Check sheet for the modelled part. Datum: model origin and axes. Units: mm. A direction names the side the tool comes from. Round coordinates to 2 decimals unless told otherwise and drop trailing zeros. Loops run counter-clockwise (first coordinate to the right, second up) from the corner with the lowest first, then second, coordinate; pieces in that order, holes last. Notation, with made-up numbers: (80, 40) - (127, 40) arc R21 ccw to (127, 64) - close; hole circle Ø2 at (-0.75, -39.75). An arc over 180 degrees is marked (long way). Return JSON: item names as keys, results as strings.
from build123d import *

# Parameters (mm, degrees)
EXTRUSION1_DEPTH = 115
ESQUISSE6_R      = 1.5
ESQUISSE6_W      = 11.044450352
ESQUISSE6_H      = 20
EXTRUSION2_DEPTH = 120


with BuildPart() as part:
    # Esquisse5 → Extrusion1 (new body)
    with BuildSketch(Plane(origin=(0, 0, 0), x_dir=(1, 0, 0), z_dir=(0, 1, 0))):
        with BuildLine():
            Line((-11.982008115, -35.006163479), (-12.953522286, -37.844501059))
            ThreePointArc((-12.953522286, -37.844501059), (-37.203278989, -14.694081546), (-35.317903714, 18.778862511))
            Line((-35.317903714, 18.778862511), (-32.669060936, 17.370447823))
            ThreePointArc((-32.669060936, 17.370447823), (-34.413033065, -13.59202543), (-11.982008115, -35.006163479))
        make_face()
    extrude(amount=EXTRUSION1_DEPTH)

    # Esquisse6 → Extrusion2 (cut)
    with BuildSketch(Plane(origin=(0, 0, 0), x_dir=(0, 0, -1), z_dir=(1, 0, 0))):
        with Locations((0, 94)):
            Circle(ESQUISSE6_R)
        with Locations((0, 87)):
            Circle(ESQUISSE6_R)
        with Locations((0, 15)):
            Circle(ESQUISSE6_R)
        with Locations((0, 22)):
            Circle(ESQUISSE6_R)
        with Locations((23.022225176, 59)):
            Rectangle(ESQUISSE6_W, ESQUISSE6_H)
    extrude(amount=-EXTRUSION2_DEPTH, mode=Mode.SUBTRACT)


solid = part.part
Q1. Tool access check on faces 1 (the face through (-12.461, 56.695, 36.405)), 2 (the face through (-34, 59, -17.5)). Record the directions out of +Z, -Z, +X, -X, +Y, -Y that give a thin tool (end or side, any length) a straight path to the whole face; none if there is none.
Answer key:
{"face 1": "+Z, +X, +Y, -Y", "face 2": "-Z, +X, -X"}
Q2. Sectioned sample at A-A (z = 0). Enter the section's corners in (x, y).
Answer key:
{"outline": "(-40, 0) - (-37, 0) - (-37, 13.5) - (-40, 13.5) - close; (-40, 16.5) - (-37, 16.5) - (-37, 20.5) - (-40, 20.5) - close; (-40, 23.5) - (-37, 23.5) - (-37, 85.5) - (-40, 85.5) - close; (-40, 88.5) - (-37, 88.5) - (-37, 92.5) - (-40, 92.5) - close; (-40, 95.5) - (-37, 95.5) - (-37, 115) - (-40, 115) - close"}
Q3. Sectioned sample at D-D (x = -28). Enter the section's corners in (y, z), plus the area to 3 significant figures.
Answer key:
{"outline": "(0, 24.19) - (115, 24.19) - (115, 28.57) - (0, 28.57) - close", "area": "504 mm²"}
Q4. Draft check along Y on faces 3 (the face through (-35, 0, 14)), 4 (the face through (-38.463, 95.487, 0.195)), 5 (the face through (-34.012, 43.917, -18.085)). Enter one of: released by +Y, released by -Y, zero draft, split by the parting line, or undercut.
Answer key:
{"face 3": "released by -Y", "face 4": "undercut", "face 5": "zero draft"}
Q5. Sectioned sample at B-B (y = 87). Enter the section's corners in (x, z), plus the area to 3 significant figures.
Answer key:
{"outline": "(-39.97, -1.5) arc R40 ccw to (-35.32, -18.78) - (-32.67, -17.37) arc R37 cw to (-36.97, -1.5) - close; (-39.97, 1.5) - (-36.97, 1.5) arc R37 cw to (-11.98, 35.01) - (-12.95, 37.84) arc R40 ccw to start", "area": "191 mm²"}
Q6. Depth check by flat-ended pin: P1, Ø2.5, axis at y = 87, z = 0, coming from the +X side (3 decimals); P2, Ø3.5, axis at y = 94, z = 0, coming from the +X side; P3, Ø10, axis at y = 62, z = -5, coming from the +X side; P4, Ø2, axis at y = 93, z = 11, coming from the -X side. Enter the tip coordinate at first touch or a pass-through.
Answer key:
{"P1": "passes through", "P2": "stops at x = -36.96", "P3": "stops at x = -35.62", "P4": "stops at x = -38.73"}
Q7. Sectioned sample at C-C (y = 53). Enter the section's corners in (x, z).
Answer key:
{"outline": "(-35.97, -17.5) - (-32.91, -17.5) - (-32.67, -17.37) arc R37 cw to (-11.98, 35.01) - (-12.95, 37.84) arc R40 ccw to start"}
Q8. Scan lines: probe 1 along Y at (x, z) = (-37.8, 0); probe 2 along Z at (x, y) = (-22, 88); probe 3 along X at (y, z) = (84, -7.5). Record each from-to range of solid material in increasing order. Write a range as [from, to].
Answer key:
{"probe 1": "y = [0, 13.5], [16.5, 20.5], [23.5, 85.5], [88.5, 92.5], [95.5, 115]", "probe 2": "z = [29.75, 33.41]", "probe 3": "x = [-39.29, -36.23]"}
